```python
from build123d import *

# Parameters (mm, degrees)
EXTRUSION1_DEPTH = 14
ESQUISSE2_R      = 1.5
EXTRUSION2_DEPTH = 39.83919024
ESQUISSE4_R      = 3
EXTRUSION3_DEPTH = 29.536760028


with BuildPart() as part:
    # Esquisse1 → Extrusion1 (new body)
    with BuildSketch(Plane.XY):
        Polygon((-31.14855853, 3.383843017), (-29.64855853, 3.383843017), (-29.64855853, -15.116156983), (-12.64855853, -15.116156983), (-12.64855853, 3.383843017), (-11.14855853, 3.383843017), (-11.14855853, -16.616156983), (-31.14855853, -16.616156983), align=None)
    extrude(amount=EXTRUSION1_DEPTH)

    # Esquisse2 → Extrusion2 (cut, through all)
    with BuildSketch(Plane(origin=(0, -15.116156983, 0), x_dir=(-1, 0, 0), z_dir=(0, 1, 0))):
        with Locations((26.14855853, 7)):
            Circle(ESQUISSE2_R)
        with Locations((16.14855853, 7)):
            Circle(ESQUISSE2_R)
    extrude(amount=-EXTRUSION2_DEPTH, mode=Mode.SUBTRACT)

    # Esquisse4 → Extrusion3 (cut, through all)
    with BuildSketch(Plane(origin=(-29.64855853, 0, 0), x_dir=(0, 0, -1), z_dir=(1, 0, 0))):
        with Locations(Location((-7, -2.616156983, 0), (0, 0, 90))):
            Circle(ESQUISSE4_R)
    extrude(amount=-EXTRUSION3_DEPTH, mode=Mode.SUBTRACT)


solid = part.part
```
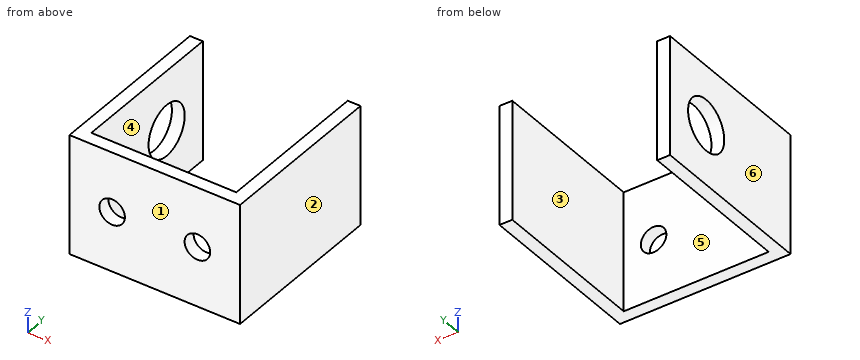
For this review, take the finished solid that the model builds, in its own axes (mm). Face numbers are marked on the shaded views. A direction names the side the tool comes from. Coordinates: 2 decimals unless noted, no trailing zeros. Order: outer loops, then holes, each group sorted by start corner. A loop starts at its lowest first (then second) coordinate and runs counter-clockwise, first axis right, second up. Notation, with made-up numbers: (30.25, -2) - (74.25, -2) arc R26 cw to (74.25, 27) - close; hole circle Ø4 at (32.5, -29.75). An arc over 180 degrees is marked (long way). Answer as a JSON object with one key per item and string values. Group by question number.
1. We need section B-B on z = 7. State the section outline as (x, y) points.
2. For the marked faces 5 and 6, list the 3-axis set-ups (+Z, -Z, +X, -X, +Y, -Y) from which the entire face can be reached by the end or side of a thin tool; tool diameter is ignored.
3. Clearance check with flat-ended pins moving along their axes: P1, Ø2.5, axis at x = -16.15, z = 7, coming from the +Y side; P2, Ø5, axis at x = -26.15, z = 7, coming from the +Y side. State where each tip first meets the part, or that it passes through.
4. The part is to be moulded in two halves that separate along X. For the marked faces 1, 2, 3 and 4, say which applies: pulls with the +X half, pulls with the -X half, needs draft (parallel to the pull), parting line crosses it, or undercut.
5. We need section D-D on y = -3.5. State the section outline as (x, z) points.
6. We need section A-A on y = 1. State the section outline as (x, z) points, then the cut area to 3 significant figures.
7. We need section C-C on z = 4.5. State the section outline as (x, y) points, then the cut area to 3 significant figures.
8. For probe 1 along X at (y, z) = (1, 6); probe 2 along Y at (x, z) = (-22.5, 10.75); probe 3 along X at (y, z) = (-3.75, 5.75), list the stretches that pass through material, from the lowest coordinate up.
Final values:
{
 "1": {"outline": "(-31.15, -16.62) - (-27.65, -16.62) - (-27.65, -15.12) - (-29.65, -15.12) - (-29.65, -5.62) - (-31.15, -5.62) - close; (-31.15, 0.38) - (-29.65, 0.38) - (-29.65, 3.38) - (-31.15, 3.38) - close; (-24.65, -16.62) - (-17.65, -16.62) - (-17.65, -15.12) - (-24.65, -15.12) - close; (-14.65, -16.62) - (-11.15, -16.62) - (-11.15, 3.38) - (-12.65, 3.38) - (-12.65, -15.12) - (-14.65, -15.12) - close"},
 "2": {"face 5": "+Z, -Z, +Y", "face 6": "+Z, -Z, -X, +Y, -Y"},
 "3": {"P1": "through", "P2": "y = -15.12"},
 "4": {"face 1": "needs draft", "face 2": "pulls with the +X half", "face 3": "undercut", "face 4": "undercut"},
 "5": {"outline": "(-31.15, 0) - (-29.65, 0) - (-29.65, 4.13) - (-31.15, 4.13) - close; (-31.15, 9.87) - (-29.65, 9.87) - (-29.65, 14) - (-31.15, 14) - close; (-12.65, 0) - (-11.15, 0) - (-11.15, 14) - (-12.65, 14) - close"},
 "6": {"outline": "(-31.15, 0) - (-29.65, 0) - (-29.65, 14) - (-31.15, 14) - close; (-12.65, 0) - (-11.15, 0) - (-11.15, 14) - (-12.65, 14) - close", "area": "42.0 mm²"},
 "7": {"outline": "(-31.15, -16.62) - (-11.15, -16.62) - (-11.15, 3.38) - (-12.65, 3.38) - (-12.65, -15.12) - (-29.65, -15.12) - (-29.65, -4.27) - (-31.15, -4.27) - close; (-31.15, -0.96) - (-29.65, -0.96) - (-29.65, 3.38) - (-31.15, 3.38) - close", "area": "80.5 mm²"},
 "8": {"probe 1": "-31.15 to -29.65, -12.65 to -11.15", "probe 2": "-16.62 to -15.12", "probe 3": "-12.65 to -11.15"}
}
